For this review, use the dimensioned drawing (mm, ordinates from the lowest corner) and the shaded views. A direction names the side the tool comes from. Coordinates: 2 decimals unless noted, no trailing zeros. Order: outer loops, then holes, each group sorted by start corner. A loop starts at its lowest first (then second) coordinate and runs counter-clockwise, first axis right, second up. Notation, with made-up numbers: (30.5, 19) -> (38.5, 19) arc R30 cw to (38.5, 44) -> close; hole circle Ø5 at (-16.5, 81.5). An arc over 180 degrees is marked (long way). Use one line per item in the form item = value. Start each with the question number.
(1) For the marked faces 1 and 2, list the 3-axis set-ups (+Z, -Z, +X, -X, +Y, -Y) from which the entire face can be reached by the end or side of a thin tool; tool diameter is ignored.
(2) Take a section at C-C (x = 19.75). State the section outline as (y, z) points (1 decimal).
(3) Take a section at A-A (z = 38.1). State how many separate pieces and enclosed holes the cut face has, then the cut area to 3 significant figures.
(4) Wall thickness on line 1 along Z through (x, y) = (23.4, 12.7); line 2 along Y through (x, z) = (11.5, 45.5) (1 decimal); line 3 along X through (y, z) = (47, 21) (1 decimal): over which ranges is each line inside the solid? List them lowest first.
(5) Mouldability with a two-part tool opening along X and no side actions: class the marked faces 3, 4, 5 and 6 as +X half, -X half, draft (parallel to the pull), parting line (faces both ways), or undercut.
(6) Take a section at D-D (x = 2). State the section outline as (y, z) points (1 decimal), then the cut area to 3 significant figures.
(7) Take a section at B-B (y = 12.7). State the section outline as (x, z) points (1 decimal).
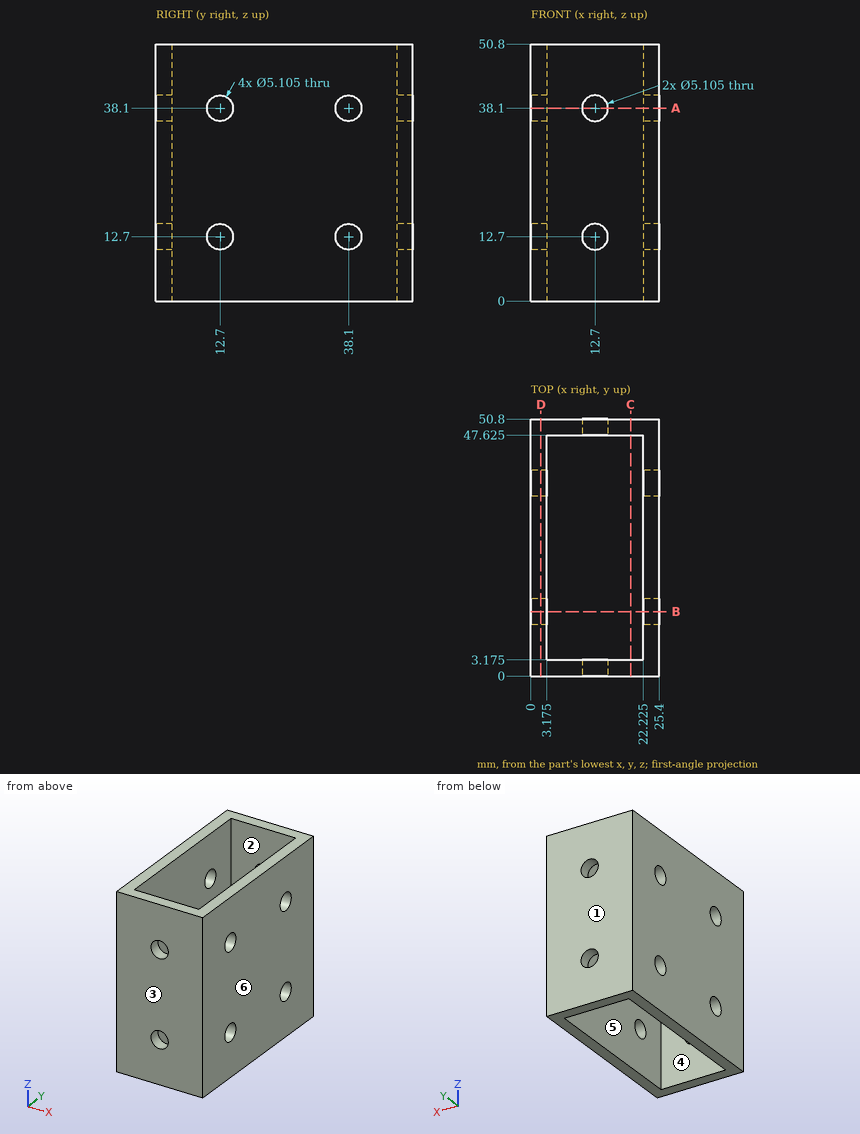
Findings:
q1.face_1 = +Z, -Z, +X, -X, +Y
q1.face_2 = +Z, -Z
q2.outline = (0, 0) -> (3.2, 0) -> (3.2, 50.8) -> (0, 50.8) -> close; (47.6, 0) -> (50.8, 0) -> (50.8, 50.8) -> (47.6, 50.8) -> close
q3.separate_pieces = 6
q3.enclosed_holes = 0
q3.area = 346 mm²
q4.line_1 = 0 to 10.15, 15.25 to 35.55, 40.65 to 50.8
q4.line_2 = 0 to 3.2, 47.6 to 50.8
q4.line_3 = 0 to 3.2, 22.2 to 25.4
q5.face_3 = draft
q5.face_4 = undercut
q5.face_5 = undercut
q5.face_6 = +X half
q6.outline = (0, 0) -> (50.8, 0) -> (50.8, 50.8) -> (0, 50.8) -> close; hole circle Ø5.1 at (12.7, 12.7); hole circle Ø5.1 at (12.7, 38.1); hole circle Ø5.1 at (38.1, 12.7); hole circle Ø5.1 at (38.1, 38.1)
q6.area = 2,500 mm²
q7.outline = (0, 0) -> (3.2, 0) -> (3.2, 10.1) -> (0, 10.1) -> close; (0, 15.3) -> (3.2, 15.3) -> (3.2, 35.5) -> (0, 35.5) -> close; (0, 40.7) -> (3.2, 40.7) -> (3.2, 50.8) -> (0, 50.8) -> close; (22.2, 0) -> (25.4, 0) -> (25.4, 10.1) -> (22.2, 10.1) -> close; (22.2, 15.3) -> (25.4, 15.3) -> (25.4, 35.5) -> (22.2, 35.5) -> close; (22.2, 40.7) -> (25.4, 40.7) -> (25.4, 50.8) -> (22.2, 50.8) -> close
